The model under review builds one solid part; all positions refer to its coordinate system, in mm. Give positions to 0.01 mm unless a question says otherwise; leave off trailing zeros. Order: outer loops, then holes, each group sorted by start corner. A loop starts at its lowest first (then second) coordinate and runs counter-clockwise, first axis right, second up. Notation, with made-up numbers: (52.25, -21) - (69.25, -21) arc R19 ccw to (69.25, -17) - close; hole circle Ø11 at (30, 50.25). An arc over 180 degrees is marked (long way). Write item = value, one per line. Start each with the question number.
1. Wall thickness on probe 1 along X at (y, z) = (-3.5, -1); probe 2 along X at (y, z) = (-5.75, 37.5); probe 3 along Z at (x, y) = (32, -5): over which ranges is each line inside the solid? List them lowest first.
2. We need section A-A, the plane z = 0. Give the boundary of the cut face in (x, y).
3. For P1, Ø6, axis at x = -38.1, z = -52.39, coming from the +Y side, flat-tipped, find the tip position at first contact; note if it passes through.
4. We need section C-C, the plane y = -4.75. State how many separate pieces and enclosed holes the cut face has, and give its area (3 significant figures).
5. We need section B-B, the plane x = 0. Give the boundary of the cut face in (y, z), and give its area (3 significant figures).
6. Mouldability with a two-part tool opening along Z and no side actions: class faces 1 (the cylindrical face through (3.7, -3.131, -16.663)), 2 (the flat face through (67.27, -3.13, 67.35)), 3 (the flat face through (69.85, -3, -1)) as pulls with the +Z half, pulls with the -Z half, needs draft (parallel to the pull), parting line crosses it, or undercut.
from build123d import *

# Parameters (mm, degrees)
F0_W     = 139.7
F0_H     = 139.7
F1_DEPTH = 6.35
F3_SIZE  = 5.08
F4_D     = 6.8
F6_D     = 6.5278
F8_D     = 34.1376


with BuildPart() as f1:
    # F0 (on Front) → F1 (new body)
    with BuildSketch(Plane.XZ):
        Rectangle(F0_W, F0_H)
    extrude(amount=F1_DEPTH)

    # F3
    f3_edges = [f1.edges().sort_by_distance(p)[0] for p in [
        (-69.85, -3.175, 69.85),
        (69.85, -3.175, 69.85),
        (69.85, -3.175, -69.85),
        (-69.85, -3.175, -69.85),
    ]]
    chamfer(f3_edges, length=F3_SIZE)

    # F4 (through all)
    with Locations(Plane(origin=(0, 0, 0), x_dir=(-1, 0, 0), z_dir=(0, 1, 0))):
        with Locations((-34.925, 34.925), (-34.925, -34.925), (34.925, -34.925), (34.925, 34.925)):
            Hole(F4_D / 2)

    # F6 (through all)
    with Locations(Plane.XZ.offset(6.35)):
        with Locations((38.1, 52.3875), (-38.1, 52.3875), (-38.1, -52.3875), (38.1, -52.3875)):
            Hole(F6_D / 2)

    # F8 (through all)
    with Locations(Plane.XZ.offset(6.35)):
        with Locations((0, 0)):
            Hole(F8_D / 2)


solid = f1.part
Model answer:
q1.probe_1 = -69.85 to -17.04, 17.04 to 69.85
q1.probe_2 = -69.85 to -37.15, -32.7 to 32.7, 37.15 to 69.85
q1.probe_3 = -69.85 to -36.66, -33.19 to 33.19, 36.66 to 69.85
q2.outline = (-69.85, -6.35) - (-17.07, -6.35) - (-17.07, 0) - (-69.85, 0) - close; (17.07, -6.35) - (69.85, -6.35) - (69.85, 0) - (17.07, 0) - close
q3.P1 = through
q4.separate_pieces = 1
q4.enclosed_holes = 9
q4.area = 18,300 mm2
q5.outline = (-6.35, -69.85) - (0, -69.85) - (0, -17.07) - (-6.35, -17.07) - close; (-6.35, 17.07) - (0, 17.07) - (0, 69.85) - (-6.35, 69.85) - close
q5.area = 670 mm2
q6.face_1 = undercut
q6.face_2 = pulls with the +Z half
q6.face_3 = needs draft
